Could you check a few things on this model? Use its own coordinates, in mm. Face numbers are marked on the shaded views. A direction names the side the tool comes from. Give positions to 0.01 mm unless a question says otherwise; leave off trailing zeros. Write each loop counter-clockwise with the first axis right and the second up, starting at its lowest first coordinate (ties: lowest second). Pieces come first, ordered by that corner, then holes. Notation, with made-up numbers: M -1,0 L 56,0 A24 ccw 56,27 Z; hole C 5.25,45 d5. An arc over 180 degrees is marked long. Use one line per item in the form item = value.
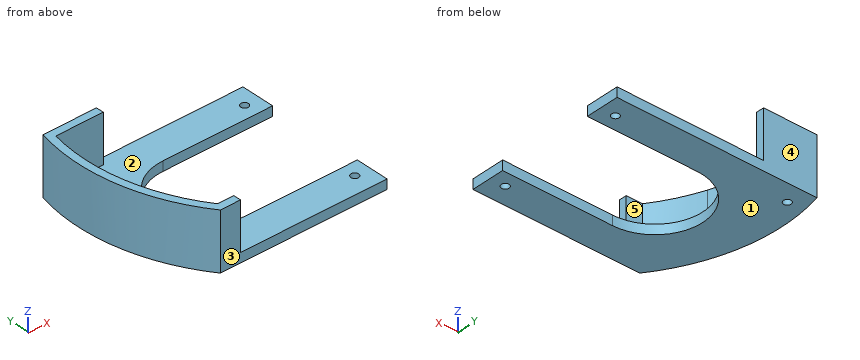
from build123d import *

# Parameters (mm, degrees)
BOSS_EXTRUDE1_DEPTH = 30
SKETCH2_R           = 2
BOSS_EXTRUDE2_DEPTH = 5


with BuildPart() as part:
    # Sketch1 → Boss-Extrude1 (new body)
    with BuildSketch(Plane.XY):
        with BuildLine():
            Line((41.601208794, 42.5), (17.731571651, 42.5))
            ThreePointArc((17.731571651, 42.5), (17.229624056, 40.505148437), (16.770533771, 38.5))
            Line((16.770533771, 38.5), (41.601208794, 38.5))
            Line((41.601208794, 38.5), (41.601208794, 42.5))
        make_face()
        with BuildLine():
            ThreePointArc((13.601208794, 42.5), (12.606987208, -1.986459129), (31.010425159, -42.5))
            Line((31.010425159, -42.5), (36.100142994, -42.5))
            ThreePointArc((36.100142994, -42.5), (34.532590926, -40.520272198), (33.017651358, -38.5))
            ThreePointArc((33.017651358, -38.5), (25.832212825, -27.03194327), (20.330809065, -14.667421089))
            ThreePointArc((20.330809065, -14.667421089), (14.78782202, 11.664315982), (16.770533771, 38.5))
            ThreePointArc((16.770533771, 38.5), (17.229624056, 40.505148437), (17.731571651, 42.5))
            Line((17.731571651, 42.5), (13.601208794, 42.5))
        make_face()
        with BuildLine():
            ThreePointArc((33.017651358, -38.5), (34.532590926, -40.520272198), (36.100142994, -42.5))
            Line((36.100142994, -42.5), (41.601208794, -42.5))
            Line((41.601208794, -42.5), (41.601208794, -38.5))
            Line((41.601208794, -38.5), (33.017651358, -38.5))
        make_face()
    extrude(amount=BOSS_EXTRUDE1_DEPTH)

    # Sketch2 → Boss-Extrude2 (add)
    with BuildSketch(Plane.XY):
        with BuildLine():
            Line((118.251926796, 42.5), (41.601208794, 42.5))
            Line((41.601208794, 42.5), (41.601208794, 38.5))
            Line((41.601208794, 38.5), (16.770533771, 38.5))
            ThreePointArc((16.770533771, 38.5), (16.641534942, -1.741302261), (33.017651358, -38.5))
            Line((33.017651358, -38.5), (41.601208794, -38.5))
            Line((41.601208794, -38.5), (41.601208794, -42.5))
            Line((41.601208794, -42.5), (118.251926796, -42.5))
            Line((118.251926796, -42.5), (118.251926796, -32.5))
            Line((118.251926796, -32.5), (118.251926796, -25))
            Line((118.251926796, -25), (60.751926796, -25))
            ThreePointArc((60.751926796, -25), (35.751926796, 0), (60.751926796, 25))
            Line((60.751926796, 25), (118.251926796, 25))
            Line((118.251926796, 25), (118.251926796, 32.5))
            Line((118.251926796, 32.5), (118.251926796, 42.5))
        make_face()
        with Locations((110.251926796, -32.5)):
            Circle(SKETCH2_R, mode=Mode.SUBTRACT)
        with Locations((20.251926796, 32.5)):
            Circle(SKETCH2_R, mode=Mode.SUBTRACT)
        with Locations((110.251926796, 32.5)):
            Circle(SKETCH2_R, mode=Mode.SUBTRACT)
    extrude(amount=BOSS_EXTRUDE2_DEPTH)


solid = part.part
1) If I drill on L1, parallel to Y at x = 37, z = 18; L2, parallel to Z at x = 23.5, y = -20.5; L3, parallel to X at y = 19, z = 14, over which ranges is the centre line in solid material (lowest first)?
Checked values:
L1 = -42.5 to -38.5, 38.5 to 42.5
L2 = 0 to 5
L3 = 10.58 to 14.58
2) I want a section at B-B, the plane y = 32.5. Please give me the cut outline in (x, z).
Checked values:
outline = M 11.62,0 L 18.25,0 L 18.25,5 L 15.66,5 L 15.66,30 L 11.62,30 Z; M 22.25,0 L 108.25,0 L 108.25,5 L 22.25,5 Z; M 112.25,0 L 118.25,0 L 118.25,5 L 112.25,5 Z
3) I want a section at A-A, the plane x = 78.5. Please give me the cut outline in (y, z), plus the area to 3 significant figures.
Checked values:
outline = M -42.5,0 L -25,0 L -25,5 L -42.5,5 Z; M 25,0 L 42.5,0 L 42.5,5 L 25,5 Z
area = 175 mm2
4) For the marked faces 4 and 5, which set-ups out of +Z, -Z, +X, -X, +Y, -Y let a thin tool reach every point of the face, with its end or its side?
Checked values:
face_4 = +Z, -Z, +X, -X, +Y
face_5 = +Z, +X
5) I want a section at D-D, the plane y = -32.5. Please give me the cut outline in (x, z), plus the area to 3 significant figures.
Checked values:
outline = M 24.31,0 L 108.25,0 L 108.25,5 L 28.98,5 L 28.98,30 L 24.31,30 Z; M 112.25,0 L 118.25,0 L 118.25,5 L 112.25,5 Z
area = 566 mm2
6) I want a section at C-C, the plane z = 26. Please give me the cut outline in (x, y).
Checked values:
outline = M 13.6,42.5 A100 ccw 31.01,-42.5 L 41.6,-42.5 L 41.6,-38.5 L 33.02,-38.5 A96 cw 16.77,38.5 L 41.6,38.5 L 41.6,42.5 Z
7) For pin 1 Ø1 at (x, y) = (78, -27) entering from -Z; pin 2 Ø5 at (x, y) = (110.25, 32.5) entering from +Z; pin 3 Ø3 at (y, z) = (-41, 12) entering from +X; pin 4 Ø4 at (y, z) = (30, 26) entering from -X, each with a flat end and sliding along its axis, tell me the tip position at first contact or that it passes through.
Checked values:
pin_1 = 0
pin_2 = 5
pin_3 = 41.6
pin_4 = 11.07
8) Thinking about a two-plate mould opening in Y: for the marked faces 1, 2 and 3, which applies, released by +Y, released by -Y, zero draft, split by the parting line, or undercut?
Checked values:
face_1 = zero draft
face_2 = undercut
face_3 = released by -Y
